```python
from build123d import *

# Parameters (mm, degrees)
SKETCH1_W           = 457.2
SKETCH1_H           = 304.8
SKETCH1_R           = 25.4
CHAMBER_BASE_DEPTH  = 6.35
SKETCH2_W           = 457.2
SKETCH2_H           = 304.8
BACK_WALL_DEPTH     = 6.35
SKETCH3_W           = 463.55
SKETCH3_H           = 457.2
SIDE_WALL_2_DEPTH   = 6.35
SKETCH5_W           = 463.55
SKETCH5_H           = 457.2
SIDE_WALL_3_DEPTH   = 6.35
SKETCH6_W           = 457.2
SKETCH6_H           = 317.5
BOSS_EXTRUDE1_DEPTH = 6.35
CUT_EXTRUDE1_DEPTH  = 6.35


with BuildPart() as part:
    # Sketch1 → Chamber Base (new body)
    with BuildSketch(Plane.XY):
        with Locations((228.6, 152.4)):
            Rectangle(SKETCH1_W, SKETCH1_H)
        with Locations((228.6, 152.4)):
            Circle(SKETCH1_R, mode=Mode.SUBTRACT)
    extrude(amount=CHAMBER_BASE_DEPTH)

    # Sketch2 → Back wall (add)
    with BuildSketch(Plane(origin=(457.2, 0, 0), x_dir=(0, 0, -1), z_dir=(1, 0, 0))):
        with Locations((-228.6, 152.4)):
            Rectangle(SKETCH2_W, SKETCH2_H)
    extrude(amount=BACK_WALL_DEPTH)

    # Sketch3 → Side wall 2 (add)
    with BuildSketch(Plane(origin=(0, 304.8, 0), x_dir=(1, 0, 0), z_dir=(0, 1, 0))):
        with Locations((231.775, -228.6)):
            Rectangle(SKETCH3_W, SKETCH3_H)
    extrude(amount=SIDE_WALL_2_DEPTH)

    # Sketch5 → Side wall 3 (add)
    with BuildSketch(Plane.XZ):
        with Locations((231.775, 228.6)):
            Rectangle(SKETCH5_W, SKETCH5_H)
    extrude(amount=SIDE_WALL_3_DEPTH)

    # Sketch6 → Boss-Extrude1 (add)
    with BuildSketch(Plane.ZY):
        with Locations((228.6, 152.4)):
            Rectangle(SKETCH6_W, SKETCH6_H)
    extrude(amount=BOSS_EXTRUDE1_DEPTH)

    # Sketch7 → Cut-Extrude1 (cut)
    with BuildSketch(Plane(origin=(0, 0, 0), x_dir=(-1, 0, 0), z_dir=(0, 0, -1))):
        with BuildLine():
            Line((-429.73498, 279.4), (-421.16502, 279.4))
            ThreePointArc((-421.16502, 279.4), (-419.704830355, 278.795169645), (-419.1, 277.33498))
            Line((-419.1, 277.33498), (-419.1, 268.76502))
            ThreePointArc((-419.1, 268.76502), (-419.704830355, 267.304830355), (-421.16502, 266.7))
            Line((-421.16502, 266.7), (-429.73498, 266.7))
            ThreePointArc((-429.73498, 266.7), (-431.195169645, 267.304830355), (-431.8, 268.76502))
            Line((-431.8, 268.76502), (-431.8, 277.33498))
            ThreePointArc((-431.8, 277.33498), (-431.195169645, 278.795169645), (-429.73498, 279.4))
        make_face()
        with BuildLine():
            Line((-38.1, 277.33498), (-38.1, 268.76502))
            ThreePointArc((-38.1, 268.76502), (-37.495169645, 267.304830355), (-36.03498, 266.7))
            Line((-36.03498, 266.7), (-27.46502, 266.7))
            ThreePointArc((-27.46502, 266.7), (-26.004830355, 267.304830355), (-25.4, 268.76502))
            Line((-25.4, 268.76502), (-25.4, 277.33498))
            ThreePointArc((-25.4, 277.33498), (-26.004830355, 278.795169645), (-27.46502, 279.4))
            Line((-27.46502, 279.4), (-36.03498, 279.4))
            ThreePointArc((-36.03498, 279.4), (-37.495169645, 278.795169645), (-38.1, 277.33498))
        make_face()
        with BuildLine():
            Line((-27.46502, 25.4), (-36.03498, 25.4))
            ThreePointArc((-36.03498, 25.4), (-37.495169645, 26.004830355), (-38.1, 27.46502))
            Line((-38.1, 27.46502), (-38.1, 36.03498))
            ThreePointArc((-38.1, 36.03498), (-37.495169645, 37.495169645), (-36.03498, 38.1))
            Line((-36.03498, 38.1), (-27.46502, 38.1))
            ThreePointArc((-27.46502, 38.1), (-26.004830355, 37.495169645), (-25.4, 36.03498))
            Line((-25.4, 36.03498), (-25.4, 27.46502))
            ThreePointArc((-25.4, 27.46502), (-26.004830355, 26.004830355), (-27.46502, 25.4))
        make_face()
        with BuildLine():
            Line((-419.1, 27.46502), (-419.1, 36.03498))
            ThreePointArc((-419.1, 36.03498), (-419.704830355, 37.495169645), (-421.16502, 38.1))
            Line((-421.16502, 38.1), (-429.73498, 38.1))
            ThreePointArc((-429.73498, 38.1), (-431.195169645, 37.495169645), (-431.8, 36.03498))
            Line((-431.8, 36.03498), (-431.8, 27.46502))
            ThreePointArc((-431.8, 27.46502), (-431.195169645, 26.004830355), (-429.73498, 25.4))
            Line((-429.73498, 25.4), (-421.16502, 25.4))
            ThreePointArc((-421.16502, 25.4), (-419.704830355, 26.004830355), (-419.1, 27.46502))
        make_face()
    extrude(amount=-CUT_EXTRUDE1_DEPTH, mode=Mode.SUBTRACT)


solid = part.part
```
For this review, take the finished solid that the model builds, in its own axes (mm). A direction names the side the tool comes from. Coordinates: 2 decimals unless noted, no trailing zeros. Order: outer loops, then holes, each group sorted by start corner. A loop starts at its lowest first (then second) coordinate and runs counter-clockwise, first axis right, second up. Notation, with made-up numbers: (32, -23) - (39, -23) arc R21 cw to (39, 11) - close; hole circle Ø11 at (13.25, 74). An arc over 180 degrees is marked (long way). Answer as a JSON object with one key per item and string values. Group by question number.
1. For faces 5 (the flat face through (457.2, 155, 235)), 6 (the flat face through (-6.35, 155, 225)), list the 3-axis set-ups (+Z, -Z, +X, -X, +Y, -Y) from which the entire face can be reached by the end or side of a thin tool; tool diameter is ignored.
2. We need section A-A on x = 228.6. State the section outline as (y, z) points.
3. We need section D-D on y = 19.5. State the section outline as (x, z) points.
4. Clearance check with a flat-ended pin moving along its axis: P1, Ø1, axis at x = 50.5, y = 42.5, coming from the +Z side. State where the tip first meets the part, or that it passes through.
5. The part is to be moulded in two halves that separate along Y. For faces 1 (the flat face through (230, -1, 457.2)), 2 (the flat face through (225, 188, 6.35)), 3 (the cylindrical face through (208.443, 136.944, 3.131)), 4 (the flat face through (232, 311.15, 225)), say which applies: pulls with the +Y half, pulls with the -Y half, needs draft (parallel to the pull), parting line crosses it, or undercut.
6. We need section B-B on y = 152.4. State the section outline as (x, z) points, then the cut area to 3 significant figures.
7. For probe 1 along Y at (x, z) = (426, 183); probe 2 along X at (y, z) = (76.5, 158); probe 3 along Y at (x, z) = (228, 1), list the stretches that pass through material, from the lowest coordinate up.
8. We need section C-C on z = 278.5. State the section outline as (x, y) points, then the cut area to 3 significant figures.
Final values:
{
 "1": {"face 5": "+Z", "face 6": "+Z, -Z, -X, +Y, -Y"},
 "2": {"outline": "(-6.35, 0) - (127, 0) - (127, 6.35) - (0, 6.35) - (0, 457.2) - (-6.35, 457.2) - close; (177.8, 0) - (311.15, 0) - (311.15, 457.2) - (304.8, 457.2) - (304.8, 6.35) - (177.8, 6.35) - close"},
 "3": {"outline": "(-6.35, 0) - (463.55, 0) - (463.55, 457.2) - (457.2, 457.2) - (457.2, 6.35) - (0, 6.35) - (0, 457.2) - (-6.35, 457.2) - close"},
 "4": {"P1": "z = 6.35"},
 "5": {"face 1": "needs draft", "face 2": "undercut", "face 3": "undercut", "face 4": "pulls with the +Y half"},
 "6": {"outline": "(-6.35, 0) - (203.2, 0) - (203.2, 6.35) - (0, 6.35) - (0, 457.2) - (-6.35, 457.2) - close; (254, 0) - (463.55, 0) - (463.55, 457.2) - (457.2, 457.2) - (457.2, 6.35) - (254, 6.35) - close", "area": "8,390 mm²"},
 "7": {"probe 1": "-6.35 to 0, 304.8 to 311.15", "probe 2": "-6.35 to 0, 457.2 to 463.55", "probe 3": "-6.35 to 127.01, 177.79 to 311.15"},
 "8": {"outline": "(-6.35, -6.35) - (463.55, -6.35) - (463.55, 311.15) - (-6.35, 311.15) - close; hole (0, 0) - (457.2, 0) - (457.2, 304.8) - (0, 304.8) - close", "area": "9,840 mm²"}
}
